Check sheet for the modelled part. Datum: model origin and axes. Units: mm. A direction names the side the tool comes from. Give positions to 0.01 mm unless a question says otherwise; leave off trailing zeros.
```python
from build123d import *

# Parameters (mm, degrees)
F2_W     = 15.24
F2_H     = 15.24
F3_DEPTH = 279.4


with BuildPart() as f1:
    # F0 (on Front) → F1 (revolve)
    with BuildSketch(Plane.XZ):
        with BuildLine():
            ThreePointArc((406.4, 50.8), (205.6655112069, 98.3292717242), (0, 114.3))
            Line((0, 114.3), (0, 96.52))
            ThreePointArc((0, 96.52), (205.7356853326, 80.3194484038), (406.4, 32.1171361113))
            Line((406.4, 32.1171361113), (406.4, 50.8))
        make_face()
        with BuildLine():
            ThreePointArc((0, 114.3), (-205.6655112069, 98.3292717242), (-406.4, 50.8))
            Line((-406.4, 50.8), (-406.4, 32.1171361113))
            ThreePointArc((-406.4, 32.1171361113), (-205.7356853326, 80.3194484038), (0, 96.52))
            Line((0, 96.52), (0, 114.3))
        make_face()
    revolve(axis=Axis((53.4217184067, 0, 0), (1, 0, 0)))

    # F2 (on face) → F3 (cut)
    with BuildSketch(Plane(origin=(-406.4, 0, 0), x_dir=(0, -1, 0), z_dir=(-1, 0, 0))):
        with BuildLine():
            Line((-7.62, 31.2000966664), (-7.62, 7.62))
            Line((-7.62, 7.62), (7.62, 7.62))
            Line((7.62, 7.62), (7.62, 31.2000966664))
            ThreePointArc((7.62, 31.2000966664), (0, 32.1171361113), (-7.62, 31.2000966664))
        make_face()
        with BuildLine():
            Line((-31.2000966664, 7.62), (-50.2252486305, 7.62))
            ThreePointArc((-50.2252486305, 7.62), (-50.8, 0), (-50.2252486305, -7.62))
            Line((-50.2252486305, -7.62), (-31.2000966664, -7.62))
            ThreePointArc((-31.2000966664, -7.62), (-32.1171361113, 0), (-31.2000966664, 7.62))
        make_face()
        with BuildLine():
            ThreePointArc((7.62, 50.2252486305), (0, 50.8), (-7.62, 50.2252486305))
            Line((-7.62, 50.2252486305), (-7.62, 31.2000966664))
            ThreePointArc((-7.62, 31.2000966664), (0, 32.1171361113), (7.62, 31.2000966664))
            Line((7.62, 31.2000966664), (7.62, 50.2252486305))
        make_face()
        with BuildLine():
            ThreePointArc((7.62, -50.2252486305), (0, -50.8), (-7.62, -50.2252486305))
            Line((-7.62, -50.2252486305), (-7.62, -127))
            Line((-7.62, -127), (7.62, -127))
            Line((7.62, -127), (7.62, -50.2252486305))
        make_face()
        with BuildLine():
            Line((7.62, -7.62), (-7.62, -7.62))
            Line((-7.62, -7.62), (-7.62, -31.2000966664))
            ThreePointArc((-7.62, -31.2000966664), (0, -32.1171361113), (7.62, -31.2000966664))
            Line((7.62, -31.2000966664), (7.62, -7.62))
        make_face()
        with BuildLine():
            Line((-7.62, -31.2000966664), (-7.62, -50.2252486305))
            ThreePointArc((-7.62, -50.2252486305), (0, -50.8), (7.62, -50.2252486305))
            Line((7.62, -50.2252486305), (7.62, -31.2000966664))
            ThreePointArc((7.62, -31.2000966664), (0, -32.1171361113), (-7.62, -31.2000966664))
        make_face()
        Rectangle(F2_W, F2_H)
        with BuildLine():
            Line((127, 7.62), (50.2252486305, 7.62))
            ThreePointArc((50.2252486305, 7.62), (50.6561083702, 3.8208225272), (50.8, 0))
            ThreePointArc((50.8, 0), (50.6561083702, -3.8208225272), (50.2252486305, -7.62))
            Line((50.2252486305, -7.62), (127, -7.62))
            Line((127, -7.62), (127, 7.62))
        make_face()
        with BuildLine():
            Line((-7.62, 7.62), (-31.2000966664, 7.62))
            ThreePointArc((-31.2000966664, 7.62), (-32.1171361113, 0), (-31.2000966664, -7.62))
            Line((-31.2000966664, -7.62), (-7.62, -7.62))
            Line((-7.62, -7.62), (-7.62, 7.62))
        make_face()
        with BuildLine():
            ThreePointArc((50.8, 0), (50.6561083702, 3.8208225272), (50.2252486305, 7.62))
            Line((50.2252486305, 7.62), (31.2000966664, 7.62))
            ThreePointArc((31.2000966664, 7.62), (31.8870521004, 3.8374914118), (32.1171361113, 0))
            ThreePointArc((32.1171361113, 0), (31.8870521004, -3.8374914118), (31.2000966664, -7.62))
            Line((31.2000966664, -7.62), (50.2252486305, -7.62))
            ThreePointArc((50.2252486305, -7.62), (50.6561083702, -3.8208225272), (50.8, 0))
        make_face()
        with BuildLine():
            Line((31.2000966664, 7.62), (7.62, 7.62))
            Line((7.62, 7.62), (7.62, -7.62))
            Line((7.62, -7.62), (31.2000966664, -7.62))
            ThreePointArc((31.2000966664, -7.62), (31.8870521004, -3.8374914118), (32.1171361113, 0))
            ThreePointArc((32.1171361113, 0), (31.8870521004, 3.8374914118), (31.2000966664, 7.62))
        make_face()
        with BuildLine():
            Line((-50.2252486305, 7.62), (-127, 7.62))
            Line((-127, 7.62), (-127, -7.62))
            Line((-127, -7.62), (-50.2252486305, -7.62))
            ThreePointArc((-50.2252486305, -7.62), (-50.8, 0), (-50.2252486305, 7.62))
        make_face()
        with BuildLine():
            Line((-7.62, 127), (-7.62, 50.2252486305))
            ThreePointArc((-7.62, 50.2252486305), (0, 50.8), (7.62, 50.2252486305))
            Line((7.62, 50.2252486305), (7.62, 127))
            Line((7.62, 127), (-7.62, 127))
        make_face()
    extrude(amount=-F3_DEPTH, mode=Mode.SUBTRACT)


solid = f1.part
```
(1) Access from +Z, -Z, +X, -X, +Y, -Y to the whole of each face (thin tool, end or side, straight path). Record for faces 1 (the face through (406.4, -1, -33)), 2 (the face through (-267, 73, -7.62)), 3 (the face through (-267, 7.62, 73)).
(2) Material ranges on line 1 (Z direction, x = 58.5, y = -49); line 2 (Z direction, x = 348.5, y = -38); line 3 (Y direction, x = 30.5, z = 9), recorded low to high.
(3) Release check for a two-part mould opening along Y. For faces 4 (the face through (-127, 0, -99)), 5 (the face through (-406.4, 29, -29)) record: pulls with the +Y half, pulls with the -Y half, needs draft (parallel to the pull), parting line crosses it, or undercut.
(4) Section check A-A on x = -328. Give the number of separate pieces and of enclosed holes in the cut face, plus the area to 3 significant figures.
(5) Gauge pin test, flat ends, axial feed: pin 1 Ø12 at (x, y) = (-61.5, -67) entering from -Z; pin 2 Ø4 at (x, y) = (52, -70) entering from -Z; pin 3 Ø12 at (y, z) = (100.5, -1.5) entering from -X. Record the tip position at first contact, or that the pin passes through.
Computed values:
1. face 1: +Z, -Z, +X, +Y, -Y
1. face 2: -X, +Y, -Y
1. face 3: +Z, -Z, -X
2. line 1: z = -101.84 to -81.64, 81.64 to 101.84
2. line 2: z = -56.28 to -31.69, 31.69 to 56.28
2. line 3: y = -113.59 to -95.74, 95.74 to 113.59
3. face 4: undercut
3. face 5: needs draft
4. separate pieces: 4
4. enclosed holes: 0
4. area: 6,270 mm2
5. pin 1: stops at z = -94.99
5. pin 2: stops at z = -90.61
5. pin 3: stops at x = -127
